Model file for the job. Use its own axes, mm. Face numbers are marked on the shaded views. A direction names the side the tool comes from. Round coordinates to 2 decimals unless told otherwise and drop trailing zeros. Order: outer loops, then holes, each group sorted by start corner. A loop starts at its lowest first (then second) coordinate and runs counter-clockwise, first axis right, second up. Notation, with made-up numbers: (34, 89.25) -> (46, 89.25) arc R21 ccw to (46, 101.25) -> close; hole circle Ø1 at (-14.75, 36.25). An arc over 180 degrees is marked (long way). Use CSV: the item, a comma, the result in double quotes.
```python
from build123d import *

# Parameters (mm, degrees)
SKETCH1_R           = 62
SKETCH2_R           = 53.5
SKETCH3_R           = 51.5
BOSS_EXTRUDE1_DEPTH = 7
SKETCH4_R           = 43.5
BOSS_EXTRUDE2_DEPTH = 7
SKETCH5_R           = 59.5
CUT_EXTRUDE1_DEPTH  = 3
SKETCH6_R           = 46
SKETCH7_R           = 36
SKETCH8_R           = 36
CUT_EXTRUDE2_DEPTH  = 92.175654809


with BuildPart() as part:
    # Sketch1 → Loft1 section 0
    with BuildSketch(Plane.XY):
        Circle(SKETCH1_R)
    # Sketch2 → Loft1 section 1
    with BuildSketch(Plane.XY.offset(27.5)):
        Circle(SKETCH2_R)
    loft()

    # Sketch3 → Boss-Extrude1 (add)
    with BuildSketch(Plane.XY.offset(27.5)):
        Circle(SKETCH3_R)
    extrude(amount=BOSS_EXTRUDE1_DEPTH)

    # Sketch4 → Boss-Extrude2 (add)
    with BuildSketch(Plane.XY.offset(34.5)):
        Circle(SKETCH4_R)
    extrude(amount=BOSS_EXTRUDE2_DEPTH)

    # Sketch5 → Cut-Extrude1 (cut)
    with BuildSketch(Plane(origin=(0, 0, 0), x_dir=(-1, 0, 0), z_dir=(0, 0, -1))):
        Circle(SKETCH5_R)
    extrude(amount=-CUT_EXTRUDE1_DEPTH, mode=Mode.SUBTRACT)

    # Sketch6 → Cut-Loft1 section 0
    with BuildSketch(Plane(origin=(0, 0, 3), x_dir=(-1, 0, 0), z_dir=(0, 0, -1))):
        Circle(SKETCH6_R)
    # Sketch7 → Cut-Loft1 section 1
    with BuildSketch(Plane(origin=(0, 0, 25), x_dir=(-1, 0, 0), z_dir=(0, 0, -1))):
        Circle(SKETCH7_R)
    loft(mode=Mode.SUBTRACT)

    # Sketch8 → Cut-Extrude2 (cut, through all)
    with BuildSketch(Plane(origin=(0, 0, 25), x_dir=(-1, 0, 0), z_dir=(0, 0, -1))):
        Circle(SKETCH8_R)
    extrude(amount=-CUT_EXTRUDE2_DEPTH, mode=Mode.SUBTRACT)


solid = part.part
```
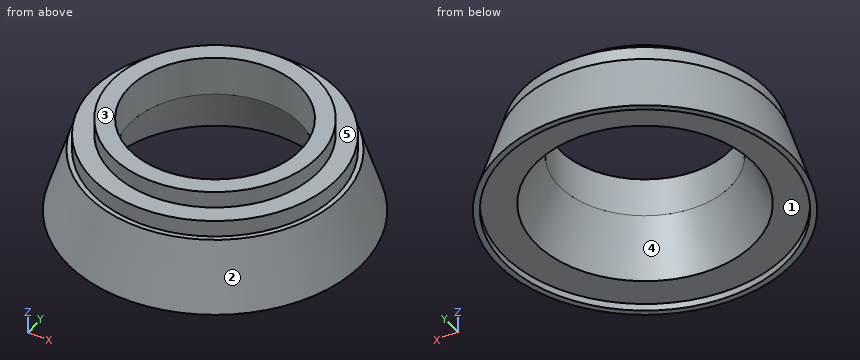
Q1. Cut at C-C (z = 9). Give the cut face in (x, y).
From the geometry:
outline,"circle Ø118.44 at (0, 0); hole circle Ø86.55 at (0, 0)"
Q2. Mould opens along Y. For the marked faces 1, 2 and 3 say: +Y half, -Y half, draft (parallel to the pull), parting line (faces both ways), or undercut.
From the geometry:
face 1,"undercut"
face 2,"parting line"
face 3,"draft"
Q3. Cut at A-A (x = 0). Give the cut face in (y, z), plus the area to 3 significant figures.
From the geometry:
outline,"(-62, 0) -> (-59.5, 0) -> (-59.5, 3) -> (-46, 3) -> (-36, 25) -> (-36, 41.5) -> (-43.5, 41.5) -> (-43.5, 34.5) -> (-51.5, 34.5) -> (-51.5, 27.5) -> (-53.5, 27.5) -> close; (36, 25) -> (46, 3) -> (59.5, 3) -> (59.5, 0) -> (62, 0) -> (53.5, 27.5) -> (51.5, 27.5) -> (51.5, 34.5) -> (43.5, 34.5) -> (43.5, 41.5) -> (36, 41.5) -> close"
area,"1,160 mm²"
Q4. Probe line 1 along Y through (x, z) = (0, 30); line 2 along X through (y, z) = (-20, 28.5); line 3 along X through (y, z) = (31, 18.5). List the from-to ranges inside material, lowest first.
From the geometry:
line 1,"y = -51.5 to -36, 36 to 51.5"
line 2,"x = -47.46 to -29.93, 29.93 to 47.46"
line 3,"x = -46.97 to -23.59, 23.59 to 46.97"
Q5. Cut at B-B (z = 37.5). Give the cut face in (x, y).
From the geometry:
outline,"circle Ø87 at (0, 0); hole circle Ø72 at (0, 0)"
Q6. Pin check, flat tips, straight feed: pin 1 (10 mm diameter, centred on x = 32.5, z = 29.5, fed in from +Y); pin 2 (4 mm diameter, centred on x = -7, z = 29, fed in from +Y); pin 3 (8 mm diameter, centred on x = 7, z = 6, fed in from -Y). Stop position of each tip, or through.
From the geometry:
pin 1,"stops at y = 45.66"
pin 2,"stops at y = 53.24"
pin 3,"stops at y = -61.05"
Q7. Which spindle directions (+Z, -Z, +X, -X, +Y, -Y) get a long thin tool onto all of the face, cutting with end or side? Do the marked faces 4 and 5. Say none if no direction does.
From the geometry:
face 4,"-Z"
face 5,"+Z"
